from build123d import *

# Parameters (mm, degrees)
ESBO_O1_W                   = 30
ESBO_O1_H                   = 45
ESBO_O1_R                   = 4.7625
RESSALTO_EXTRUS_O1_DEPTH    = 12
FURO_COM_FOLGA_DE_M31_D     = 3.6
FURO_COM_FOLGA_DE_M31_DEPTH = 30
FURO_COM_FOLGA_DE_M31_TIP   = 1.081549114


with BuildPart() as part:
    # Esboço1 → Ressalto-extrusão1 (new body)
    with BuildSketch(Plane.XY.offset(-196.305879913)):
        with Locations((18.764782864, 16.732361179)):
            Rectangle(ESBO_O1_W, ESBO_O1_H)
        with Locations((18.764782864, 30.002354844)):
            Circle(ESBO_O1_R, mode=Mode.SUBTRACT)
        with Locations((18.764782864, 4.232361179)):
            Circle(ESBO_O1_R, mode=Mode.SUBTRACT)
    extrude(amount=RESSALTO_EXTRUS_O1_DEPTH)

    # Furo com folga de M31
    with Locations(Plane.ZY.offset(-3.764782864)):
        with Locations((-189.305879913, 30.002361179), (-189.305879913, 4.232361179)):
            Hole(FURO_COM_FOLGA_DE_M31_D / 2, depth=FURO_COM_FOLGA_DE_M31_DEPTH)
            with Locations((0, 0, -(FURO_COM_FOLGA_DE_M31_DEPTH + FURO_COM_FOLGA_DE_M31_TIP / 2))):  # 118° drill point
                Cone(0, FURO_COM_FOLGA_DE_M31_D / 2, FURO_COM_FOLGA_DE_M31_TIP, mode=Mode.SUBTRACT)


solid = part.part
The model under review builds one solid part; all positions refer to its coordinate system, in mm. Coordinates: 2 decimals unless noted, no trailing zeros. Loops run counter-clockwise (first coordinate to the right, second up) from the corner with the lowest first, then second, coordinate; pieces in that order, holes last. Notation, with made-up numbers: M -18.5,-12.5 L 3.5,-12.5 A15 ccw 3.5,-2.5 Z; hole C 80.25,88.5 d7. An arc over 180 degrees is marked long. Put each result on its own line as item: value. Start each with the question number.
Q1. Add section A-A (x = 22). Write out the cut boundary in (y, z).
Q2. Add section C-C (y = 3). Write out the cut boundary in (x, z), and give its area (3 significant figures).
Q3. Add section B-B (y = 26.5). Write out the cut boundary in (x, z), and give its area (3 significant figures).
Q4. Wall thickness on line 1 (Y direction, x = 18.5, z = -188.75); line 2 (Y direction, x = 11, z = -188.75); line 3 (X direction, y = 2.5, z = -186): over which ranges is each line inside the solid? List them lowest first.
Q5. The part is to be moulded in two halves that separate along Y. For faces 1 (the cylindrical face through (9.135, 30.082, -187.508)), 2 (the flat face through (33.765, 16, -190)), 3 (the flat face through (19, 39.232, -190)), say which applies: +Y half, -Y half, draft (parallel to the pull), parting line (faces both ways), or undercut.
Q6. Add section D-D (z = -190.25). Write out the cut boundary in (x, y) (1 decimal), and give its area (3 significant figures).
Answers:
1. outline: M -5.77,-196.31 L 0.74,-196.31 L 0.74,-184.31 L -5.77,-184.31 Z; M 7.73,-196.31 L 26.51,-196.31 L 26.51,-184.31 L 7.73,-184.31 Z; M 33.5,-196.31 L 39.23,-196.31 L 39.23,-184.31 L 33.5,-184.31 Z
2. outline: M 3.76,-196.31 L 14.16,-196.31 L 14.16,-190.62 L 3.76,-190.62 Z; M 3.76,-187.99 L 14.16,-187.99 L 14.16,-184.31 L 3.76,-184.31 Z; M 23.37,-196.31 L 33.76,-196.31 L 33.76,-190.62 L 23.37,-190.62 Z; M 23.37,-187.99 L 33.76,-187.99 L 33.76,-184.31 L 23.37,-184.31 Z
2. area: 195 mm^2
3. outline: M 3.76,-196.31 L 15.54,-196.31 L 15.54,-184.31 L 3.76,-184.31 Z; M 21.99,-196.31 L 33.76,-196.31 L 33.76,-184.31 L 21.99,-184.31 Z
3. area: 283 mm^2
4. line 1: y = -5.77 to -0.52, 8.99 to 25.25, 34.76 to 39.23
4. line 2: y = -5.77 to 2.52, 5.94 to 28.29, 31.71 to 39.23
4. line 3: x = 3.76 to 14.33, 23.2 to 33.76
5. face 1: undercut
5. face 2: draft
5. face 3: +Y half
6. outline: M 3.8,-5.8 L 33.8,-5.8 L 33.8,2.7 L 23.3,2.7 A4.8 cw 14.3,2.7 L 3.8,2.7 Z; M 3.8,5.8 L 14.3,5.8 A4.8 cw 23.3,5.8 L 33.8,5.8 L 33.8,28.5 L 23.3,28.5 A4.8 cw 14.3,28.5 L 3.8,28.5 Z; M 3.8,31.5 L 14.3,31.5 A4.8 cw 23.3,31.5 L 33.8,31.5 L 33.8,39.2 L 3.8,39.2 Z
6. area: 1,080 mm^2
